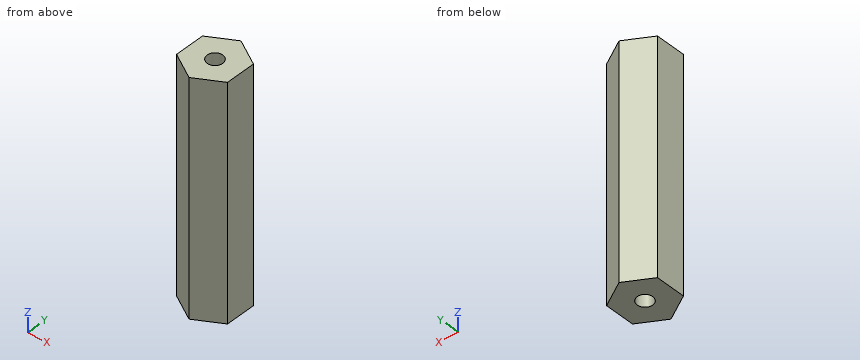
Autodesk Inventor part; units mm, degrees
ref_plane "YZ Plane" through (0, 0, 0) normal (1, 0, 0) x (0, 1, 0)
ref_plane "XZ Plane" through (0, 0, 0) normal (0, 1, 0) x (-1, 0, 0)
ref_plane "XY Plane" through (0, 0, 0) normal (0, 0, 1) x (1, 0, 0)
sketch "Sketch1" plane through (0, 0, 0) normal (0, 0, 1) x (1, 0, 0)
  circle A0 centre (0, 0) radius 0.9 construction
  circle A1 centre (0, 0) radius 3.3 construction
  line L0 (3.3, -1.9053) -> (0, -3.8105)
  line L1 (0, -3.8105) -> (-3.3, -1.9053)
  line L2 (-3.3, -1.9053) -> (-3.3, 1.9053)
  line L3 (-3.3, 1.9053) -> (0, 3.8105)
  line L4 (0, 3.8105) -> (3.3, 1.9053)
  line L5 (3.3, 1.9053) -> (3.3, -1.9053)
  circle A2 centre (0, 0) radius 0.6
  point P0 (3.3, 0)
  dimension "d0" = 1.8
  dimension "d1" = 2.4
  dimension "d4" = 1.2
extrude "Extrusion1" add sketch "Sketch1" along normal blind 30
sketch "Sketch2" plane through (0, 0, 0) normal (0, 0, -1) x (-1, 0, 0)
  circle A0 centre (0, 0) radius 0.6
hole "Hole1" at (0, 0, 0) direction (0, 0, 1) diameter 2 end through all
properties part number "Standoff_V1"
Here's how the part is built. I have some questions about the finished solid (model axes, mm). Round coordinates to 2 decimals unless told otherwise and drop trailing zeros. Loops run counter-clockwise (first coordinate to the right, second up) from the corner with the lowest first, then second, coordinate; pieces in that order, holes last. Notation, with made-up numbers: (88.5, 18.25) -> (102.5, 18.25) arc R21 ccw to (102.5, 26.25) -> close; hole circle Ø6 at (61, 43). An arc over 180 degrees is marked (long way). Write each question's results on one line, items separated by ' | '.
(1) If I drill on L1, parallel to X at y = 0, z = 11.5; L2, parallel to X at y = -0.5, z = 20.75; L3, parallel to Y at x = -2, z = 18, over which ranges is the centre line in solid material (lowest first)?
Worked answers:
L1: -3.3 to -1, 1 to 3.3 | L2: -3.3 to -0.87, 0.87 to 3.3 | L3: -2.66 to 2.66
(2) If we section it at B-B, the plane z = 2.5: List the corners of the cut face in (x, y) for me, then the cut area to 3 significant figures.
Worked answers:
outline: (-3.3, -1.91) -> (0, -3.81) -> (3.3, -1.91) -> (3.3, 1.91) -> (0, 3.81) -> (-3.3, 1.91) -> close; hole circle Ø2 at (0, 0) | area: 34.6 mm2
(3) If we section it at C-C, the plane x = -2.5: List the corners of the cut face in (y, z) for me.
Worked answers:
outline: (-2.37, 0) -> (2.37, 0) -> (2.37, 30) -> (-2.37, 30) -> close
(4) For P1, Ø1.5, axis at x = 2.5, z = 18.5, coming from the +Y side; P2, Ø2, axis at y = 2.5, z = 13, coming from the +X side, each with a flat end and sliding along its axis, tell me the tip position at first contact or that it passes through.
Worked answers:
P1: y = 2.8 | P2: x = 3.3
(5) If we section it at D-D, the plane y = -3: List the corners of the cut face in (x, z) for me, then the cut area to 3 significant figures.
Worked answers:
outline: (-1.4, 0) -> (1.4, 0) -> (1.4, 30) -> (-1.4, 30) -> close | area: 84.2 mm2
(6) If we section it at A-A, the plane y = 0: List the corners of the cut face in (x, z) for me, then the cut area to 3 significant figures.
Worked answers:
outline: (-3.3, 0) -> (-1, 0) -> (-1, 30) -> (-3.3, 30) -> close; (1, 0) -> (3.3, 0) -> (3.3, 30) -> (1, 30) -> close | area: 138 mm2
